Here's how the part is built. I have some questions about the finished solid (model axes, mm). A direction names the side the tool comes from. Give positions to 0.01 mm unless a question says otherwise; leave off trailing zeros. Order: outer loops, then holes, each group sorted by start corner. A loop starts at its lowest first (then second) coordinate and runs counter-clockwise, first axis right, second up.
from build123d import *

# Parameters (mm, degrees)
BOSS_EXTRUDE4_DEPTH = 12.7
CUT_EXTRUDE4_DEPTH  = 12.7
SKETCH13_W          = 6.35
SKETCH13_H          = 0.762
CUT_EXTRUDE5_DEPTH  = 12.7
LPATTERN3_COUNT     = 12
LPATTERN3_PITCH     = 14.9733
SKETCH14_W          = 6.35
SKETCH14_H          = 0.762
CUT_EXTRUDE6_DEPTH  = 12.7
LPATTERN4_COUNT     = 12
LPATTERN4_PITCH     = 14.9733


with BuildPart() as part:
    # Sketch11 → Boss-Extrude4 (new body)
    with BuildSketch(Plane.XY):
        with BuildLine():
            Line((-84.8995, 31.75), (84.8995, 31.75))
            ThreePointArc((84.8995, 31.75), (116.6495, 0), (84.8995, -31.75))
            Line((84.8995, -31.75), (-84.8995, -31.75))
            ThreePointArc((-84.8995, -31.75), (-116.6495, 0), (-84.8995, 31.75))
        make_face()
    extrude(amount=BOSS_EXTRUDE4_DEPTH)

    # Sketch12 → Cut-Extrude4 (cut)
    with BuildSketch(Plane.XY.offset(12.7)):
        with BuildLine():
            Line((-83.312, 30.1625), (83.312, 30.1625))
            ThreePointArc((83.312, 30.1625), (113.4745, 0), (83.312, -30.1625))
            Line((83.312, -30.1625), (-83.312, -30.1625))
            ThreePointArc((-83.312, -30.1625), (-113.4745, 0), (-83.312, 30.1625))
        make_face()
    extrude(amount=-CUT_EXTRUDE4_DEPTH, mode=Mode.SUBTRACT)

    # Sketch13 → Cut-Extrude5 (cut)
    with BuildSketch(Plane(origin=(0, 0, 0), x_dir=(-1, 0, 0), z_dir=(0, 0, -1))):
        with Locations((-81.7245, 31.369)):
            Rectangle(SKETCH13_W, SKETCH13_H)
    cut_extrude5 = extrude(amount=-CUT_EXTRUDE5_DEPTH, mode=Mode.SUBTRACT)

    # LPattern3: Cut-Extrude5 ×12
    with Locations(*[(-i * LPATTERN3_PITCH, 0, 0) for i in range(1, LPATTERN3_COUNT)]):
        add(cut_extrude5, mode=Mode.SUBTRACT)

    # Sketch14 → Cut-Extrude6 (cut)
    with BuildSketch(Plane(origin=(0, 0, 0), x_dir=(-1, 0, 0), z_dir=(0, 0, -1))):
        with Locations((-81.7245, -31.369)):
            Rectangle(SKETCH14_W, SKETCH14_H)
    cut_extrude6 = extrude(amount=-CUT_EXTRUDE6_DEPTH, mode=Mode.SUBTRACT)

    # LPattern4: Cut-Extrude6 ×12
    with Locations(*[(-i * LPATTERN4_PITCH, 0, 0) for i in range(1, LPATTERN4_COUNT)]):
        add(cut_extrude6, mode=Mode.SUBTRACT)


solid = part.part
Q1. I'm going to push flat-ended pins straight in: P1, Ø1.9, axis at x = 51.5, z = 6, coming from the -Y side; P2, Ø6, axis at x = -83.5, z = 3, coming from the -Y side; P3, Ø5, axis at x = -38.5, z = 5.5, coming from the +Y side. Where does each tip first touch, or does it pass through?
Filled sheet:
P1: stops at y = -30.99
P2: stops at y = -31.73
P3: stops at y = 30.99
Q2. I need wall thicknesses on L1, parallel to Y at x = 43, z = 5.75; L2, parallel to X at y = -0.5, z = 8.5; L3, parallel to Y at x = -39, z = 4.5. Which ranges of each line are inside material? Lowest first, please.
Filled sheet:
L1: y = -31.75 to -30.16, 30.16 to 31.75
L2: x = -116.65 to -113.47, 113.47 to 116.65
L3: y = -30.99 to -30.16, 30.16 to 30.99
Q3. For faces 1 (the face through (37, 30.988, 6)), 2 (the face through (-68, -30.988, 6)), 3 (the face through (-60, -31.75, 6)), which set-ups out of +Z, -Z, +X, -X, +Y, -Y let a thin tool reach every point of the face, with its end or its side?
Filled sheet:
face 1: +Z, -Z, +Y
face 2: +Z, -Z, -Y
face 3: +Z, -Z, +X, -X, -Y
Q4. If we section it at A-A on y = 0: List the corners of the cut face in (x, z) for me.
Filled sheet:
outline: (-116.65, 0) - (-113.47, 0) - (-113.47, 12.7) - (-116.65, 12.7) - close; (113.47, 0) - (116.65, 0) - (116.65, 12.7) - (113.47, 12.7) - close
Q5. If we section it at B-B on x = 30: List the corners of the cut face in (y, z) for me, plus the area to 3 significant figures.
Filled sheet:
outline: (-31.75, 0) - (-30.16, 0) - (-30.16, 12.7) - (-31.75, 12.7) - close; (30.16, 0) - (31.75, 0) - (31.75, 12.7) - (30.16, 12.7) - close
area: 40.3 mm2
Q6. Thinking about a two-plate mould opening in X: for faces 4 (the face through (-46, 31.75, 6)), 5 (the face through (113.467, 0.663, 6.439)), which applies, released by +X, released by -X, zero draft, split by the parting line, or undercut?
Filled sheet:
face 4: zero draft
face 5: undercut
